Part model, mm, in its own coordinate system. Face numbers are marked on the shaded views. A direction names the side the tool comes from. Give positions to 0.01 mm unless a question says otherwise; leave off trailing zeros. Order: outer loops, then holes, each group sorted by start corner. A loop starts at its lowest first (then second) coordinate and runs counter-clockwise, first axis right, second up. Notation, with made-up numbers: (87, 29) - (127, 29) arc R14 ccw to (127, 39) - close; hole circle Ø10 at (-18, 23). An arc over 180 degrees is marked (long way). Use a Markdown table: item, result. Add a question column.
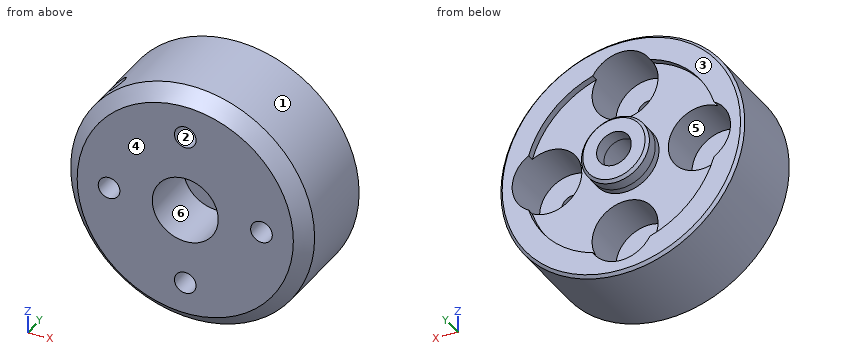
from build123d import *

# Parameters (mm, degrees)
SKETCH2_R                 = 11.176
BOSS_EXTRUDE1_DEPTH       = 9.144
SKETCH3_R                 = 8.89
SKETCH3_R_2               = 3.1115
CUT_EXTRUDE1_DEPTH        = 0.635
SKETCH4_R                 = 3.0226
CUT_EXTRUDE2_DEPTH        = 5.334
SKETCH6_R                 = 3.0226
CUT_EXTRUDE4_DEPTH        = 4.699
CIRPATTERN5_COUNT         = 4
SKETCH7_R                 = 1.5875
CUT_EXTRUDE5_DEPTH        = 8.255
CHAMFER1_SIZE             = 0.254
CHAMFER2_SIZE             = 1.27
SKETCH8_R                 = 0.9921875
CUT_EXTRUDE6_DEPTH        = 4.445
CIRPATTERN6_COUNT         = 4
SKETCH10_R                = 3.1115
SKETCH10_R_2              = 1.5875
BOSS_EXTRUDE2_DEPTH       = 1.27
CHAMFER3_SIZE             = 0.254
F_2_56_TAPPED_HOLE3_D     = 1.778
F_2_56_TAPPED_HOLE3_DEPTH = 11.43
F_2_56_TAPPED_HOLE3_TIP   = 0.53416509


with BuildPart() as part:
    # Sketch2 → Boss-Extrude1 (new body)
    with BuildSketch(Plane(origin=(0, 0, 0), x_dir=(1, 0, 0), z_dir=(0, 1, 0))):
        Circle(SKETCH2_R)
    extrude(amount=BOSS_EXTRUDE1_DEPTH)

    # Sketch3 → Cut-Extrude1 (cut)
    with BuildSketch(Plane(origin=(0, 9.144, 0), x_dir=(1, 0, 0), z_dir=(0, 1, 0))):
        Circle(SKETCH3_R)
        Circle(SKETCH3_R_2, mode=Mode.SUBTRACT)
    extrude(amount=-CUT_EXTRUDE1_DEPTH, mode=Mode.SUBTRACT)

    # Sketch4 → Cut-Extrude2 (cut)
    with BuildSketch(Plane(origin=(0, 0, 0), x_dir=(-1, 0, 0), z_dir=(0, -1, 0))):
        Circle(SKETCH4_R)
    extrude(amount=-CUT_EXTRUDE2_DEPTH, mode=Mode.SUBTRACT)

    # Sketch6 → Cut-Extrude4 (cut)
    with BuildSketch(Plane(origin=(0, 9.144, 0), x_dir=(1, 0, 0), z_dir=(0, 1, 0))):
        with Locations((0, 6.985)):
            Circle(SKETCH6_R)
    cut_extrude4 = extrude(amount=-CUT_EXTRUDE4_DEPTH, mode=Mode.SUBTRACT)

    # CirPattern5: Cut-Extrude4 ×4 about axis
    cirpattern5_axis = Axis((0, 0, 0), (0, 1, 0))
    for i in range(1, CIRPATTERN5_COUNT):
        add(cut_extrude4.rotate(cirpattern5_axis, i * 360 / CIRPATTERN5_COUNT), mode=Mode.SUBTRACT)

    # Sketch7 → Cut-Extrude5 (cut)
    with BuildSketch(Plane(origin=(0, 9.144, 0), x_dir=(1, 0, 0), z_dir=(0, 1, 0))):
        Circle(SKETCH7_R)
    extrude(amount=-CUT_EXTRUDE5_DEPTH, mode=Mode.SUBTRACT)

    # Chamfer1
    chamfer1_edges = [part.edges().sort_by_distance(p)[0] for p in [
        (-11.176, 9.144, 0),
    ]]
    chamfer(chamfer1_edges, length=CHAMFER1_SIZE)

    # Chamfer2
    chamfer2_edges = [part.edges().sort_by_distance(p)[0] for p in [
        (-11.176, 0, 0),
    ]]
    chamfer(chamfer2_edges, length=CHAMFER2_SIZE)

    # Sketch8 → Cut-Extrude6 (cut)
    with BuildSketch(Plane(origin=(0, 4.445, 0), x_dir=(1, 0, 0), z_dir=(0, 1, 0))):
        with Locations((0, 6.985)):
            Circle(SKETCH8_R)
    cut_extrude6 = extrude(amount=-CUT_EXTRUDE6_DEPTH, mode=Mode.SUBTRACT)

    # CirPattern6: Cut-Extrude6 ×4 about axis
    cirpattern6_axis = Axis((0, 0, 0), (0, 1, 0))
    for i in range(1, CIRPATTERN6_COUNT):
        add(cut_extrude6.rotate(cirpattern6_axis, i * 360 / CIRPATTERN6_COUNT), mode=Mode.SUBTRACT)

    # Sketch10 → Boss-Extrude2 (add)
    with BuildSketch(Plane(origin=(0, 9.144, 0), x_dir=(1, 0, 0), z_dir=(0, 1, 0))):
        Circle(SKETCH10_R)
        Circle(SKETCH10_R_2, mode=Mode.SUBTRACT)
    extrude(amount=BOSS_EXTRUDE2_DEPTH)

    # Chamfer3
    chamfer3_edges = [part.edges().sort_by_distance(p)[0] for p in [
        (-3.1115, 10.414, 0),
    ]]
    chamfer(chamfer3_edges, length=CHAMFER3_SIZE)

    # 2-56 Tapped Hole3
    with Locations(Plane(origin=(-8.082230509, 0, 8.082230509), x_dir=(0, -1, 0), z_dir=(-0.707106781, 0, 0.707106781))):
        with Locations((-3.175, 0)):
            Hole(F_2_56_TAPPED_HOLE3_D / 2, depth=F_2_56_TAPPED_HOLE3_DEPTH)
            with Locations((0, 0, -(F_2_56_TAPPED_HOLE3_DEPTH + F_2_56_TAPPED_HOLE3_TIP / 2))):  # 118° drill point
                Cone(0, F_2_56_TAPPED_HOLE3_D / 2, F_2_56_TAPPED_HOLE3_TIP, mode=Mode.SUBTRACT)


solid = part.part
1. Tool access for the marked faces 4, 5 and 6: list every direction of +Z, -Z, +X, -X, +Y, -Y with a clear straight run to the whole face (end or side of a thin tool).
2. Pin check, flat tips, straight feed: P1, Ø8, axis at x = 0, z = -6.985, coming from the +Y side; P2, Ø2, axis at x = 7.5, y = 8, coming from the +Z side; P3, Ø3, axis at x = 1, z = -8, coming from the +Y side (3 decimals); P4, Ø6.5, axis at x = -3, z = -2, coming from the +Y side. Stop position of each tip, or through.
3. Cut at B-B (y = 9.5). Write the cut outline in (x, z) (1 decimal), plus the area to 3 significant figures.
4. Drill centre lines: probe 1 along Z at (x, y) = (0, 8.1); probe 2 along X at (y, z) = (3.65, 0). Where is each one in solid material? Low to high. Write a range as [from, to].
5. Mould opens along Z. For the marked faces 1, 2 and 3 say: released by +Z, released by -Z, zero draft, split by the parting line, or undercut.
6. Cut at D-D (y = 3.5). Write the cut outline in (x, z) (3 decimals), plus the area to 3 significant figures.
7. Cut at A-A (z = 0). State how many separate pieces and enclosed holes the cut face has, plus the area to 3 significant figures.
Responses:
| question | item | result |
|---|---|---|
| 1 | face 4 | +Z, -Z, +X, -X, -Y |
| 1 | face 5 | +Y |
| 1 | face 6 | -Y |
| 2 | P1 | stops at y = 10.29 |
| 2 | P2 | stops at z = 9.09 |
| 2 | P3 | stops at y = 4.445 |
| 2 | P4 | stops at y = 10.41 |
| 3 | outline | circle Ø6.2 at (0, 0); hole circle Ø3.2 at (0, 0) |
| 3 | area | 22.5 mm² |
| 4 | probe 1 | z = [-11.18, -10.01], [-3.96, -1.59], [1.59, 3.96], [10.01, 11.18] |
| 4 | probe 2 | x = [-11.18, -7.98], [-5.99, -3.02], [3.02, 5.99], [7.98, 11.18] |
| 5 | face 1 | split by the parting line |
| 5 | face 2 | undercut |
| 5 | face 3 | zero draft |
| 6 | outline | (-8.466, 7.296) arc R11.176 ccw (long way) to (-7.296, 8.466) - (-1.471, 2.641) arc R3.023 cw (long way) to (-2.641, 1.471) - close; hole circle Ø1.984 at (-6.985, 0); hole circle Ø1.984 at (0, -6.985); hole circle Ø1.984 at (0, 6.985); hole circle Ø1.984 at (6.985, 0) |
| 6 | area | 338 mm² |
| 7 | separate pieces | 4 |
| 7 | enclosed holes | 0 |
| 7 | area | 86.6 mm² |
